The figure shows three views and two pictorial views of one solid part (mm, origin at its lowest corner). Answer the questions. Coordinates: 2 decimals unless noted, no trailing zeros. Order: outer loops, then holes, each group sorted by start corner. A loop starts at its lowest first (then second) coordinate and runs counter-clockwise, first axis right, second up. Notation, with made-up numbers: M 40,89 L 49,89 A20 cw 49,121 Z; hole C -12,53 d1. An arc over 180 degrees is marked long. Answer in a Markdown table with one row per item. Add a question column.
Item 1: Flat-ended cylindrical pins translate along their axes: pin 1 Ø4 at (x, y) = (333, 6.5) entering from +Z; pin 2 Ø3 at (y, z) = (1.5, 251.5) entering from -X; pin 3 Ø6.5 at (x, y) = (7.5, 6.5) entering from -Z. Find the tip coordinate at first contact, or state that the pin passes through.
Item 2: The part is cut by section B-B (z = 153.5). Write down the section's boundary in (x, y), then the cut area to 3 significant figures.
Item 3: The part is cut by section A-A (x = 320). Write down the section's boundary in (y, z).
Item 4: The part is cut by section C-C (z = 232). Write down the section's boundary in (x, y).
Item 5: Consider line 1 (Z direction, x = 183.5, y = 5.5); line 2 (Z direction, x = 320, y = 9.5); line 3 (X direction, y = 2.75, z = 227). Determine where each line is inside the solid, lowest interval first. Write a range as from..to.
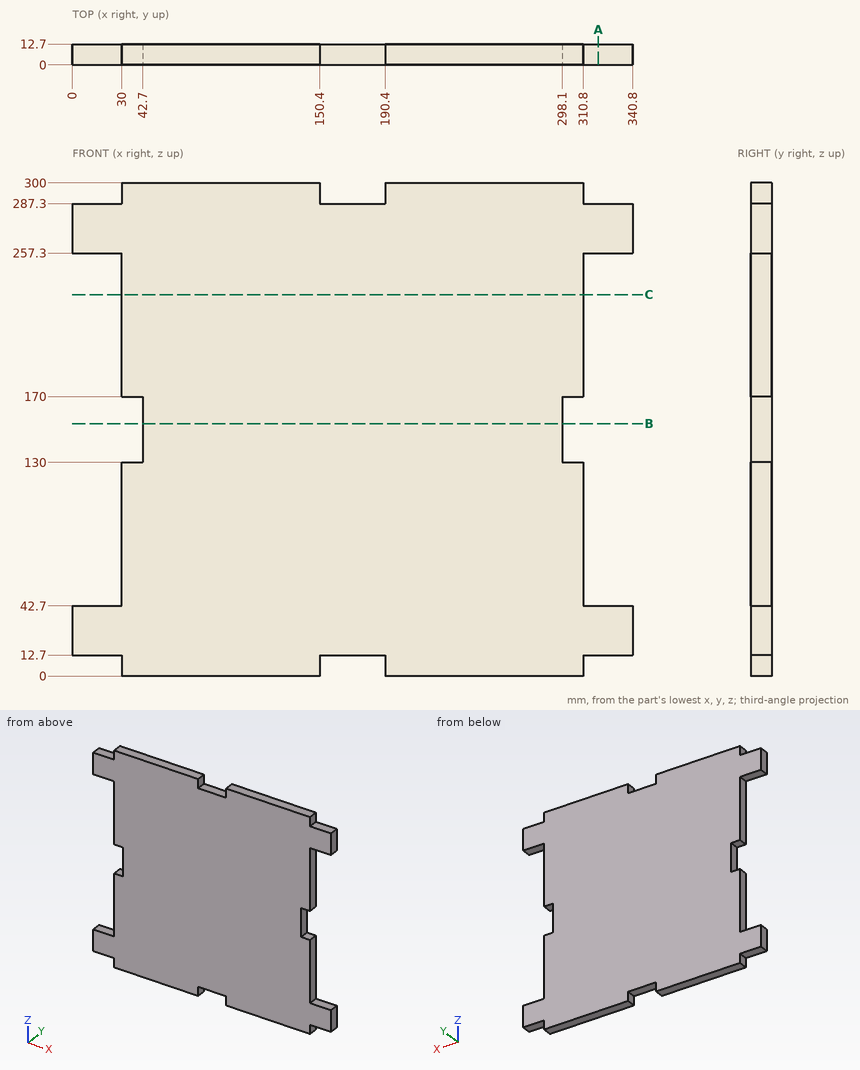
Reply:
| question | item | result |
|---|---|---|
| 1 | pin 1 | stops at z = 287.3 |
| 1 | pin 2 | stops at x = 30 |
| 1 | pin 3 | stops at z = 12.7 |
| 2 | outline | M 42.7,0 L 298.1,0 L 298.1,12.7 L 42.7,12.7 Z |
| 2 | area | 3,240 mm2 |
| 3 | outline | M 0,12.7 L 12.7,12.7 L 12.7,42.7 L 0,42.7 Z; M 0,257.3 L 12.7,257.3 L 12.7,287.3 L 0,287.3 Z |
| 4 | outline | M 30,0 L 310.8,0 L 310.8,12.7 L 30,12.7 Z |
| 5 | line 1 | z = 12.7..287.3 |
| 5 | line 2 | z = 12.7..42.7, 257.3..287.3 |
| 5 | line 3 | x = 30..310.8 |
